```python
from build123d import *

# Parameters (mm, degrees)
SKETCH1_R                = 19.939
CIRCLE_EXTRUDE_DEPTH     = 6.35
SKETCH3_W                = 6.35
SKETCH3_H                = 39.878
RECTANGLE_EXTRUDE_DEPTH  = 127
SKETCH2_R                = 18.034
CIRCLE_CUT_DEPTH         = 129.712416732
SKETCH6_W                = 125.095
SKETCH6_H                = 36.068
RECTANGLE_CUT_DEPTH      = 129.712416732
SKETCH7_W                = 61.595
SKETCH7_H                = 36.068
END_SHAPE_DEPTH          = 6.35
SKETCH8_R                = 1.905
FOR_SPRING_EXTRUDE_DEPTH = 2.54
MIRRORED_PATTERN_COUNT   = 2
MIRRORED_PATTERN_PITCH   = 254
MIDDLE_CONNECTOR_REACH   = 256.861
SKETCH10_W               = 6.35
SKETCH10_H               = 39.878
SKETCH11_W               = 6.35
SKETCH11_H               = 39.878
END_CUT_DEPTH            = 55.88


with BuildPart() as part:
    # Sketch1 → circle extrude (new body)
    with BuildSketch(Plane.XY):
        Circle(SKETCH1_R)
    extrude(amount=CIRCLE_EXTRUDE_DEPTH)

    # Sketch3 → rectangle extrude (add)
    with BuildSketch(Plane(origin=(0, 0, 0), x_dir=(0, 0, -1), z_dir=(1, 0, 0))):
        with Locations((-3.175, 0)):
            Rectangle(SKETCH3_W, SKETCH3_H)
    extrude(amount=RECTANGLE_EXTRUDE_DEPTH)

    # Sketch2 → circle cut (cut, through all)
    with BuildSketch(Plane.XY.offset(6.35)):
        Circle(SKETCH2_R)
    extrude(amount=-CIRCLE_CUT_DEPTH, mode=Mode.SUBTRACT)

    # Sketch6 → rectangle cut (cut, through all)
    with BuildSketch(Plane.XY.offset(6.35)):
        with Locations((62.5475, 0)):
            Rectangle(SKETCH6_W, SKETCH6_H)
    extrude(amount=-RECTANGLE_CUT_DEPTH, mode=Mode.SUBTRACT)

    # Sketch7 → end shape (add)
    with BuildSketch(Plane.XY.offset(6.35)):
        with Locations((94.2975, 0)):
            Rectangle(SKETCH7_W, SKETCH7_H)
    extrude(amount=-END_SHAPE_DEPTH)

    # Sketch8 → for spring extrude (add)
    with BuildSketch(Plane.ZY.offset(-63.5)):
        with Locations((3.175, 0)):
            Circle(SKETCH8_R)
    extrude(amount=FOR_SPRING_EXTRUDE_DEPTH)


with BuildPart() as mirrored_pattern_1:
    # mirrored pattern: pattern copy
    add(part.part.moved(Location(Vector(1, 0, 0) * (1 * MIRRORED_PATTERN_PITCH))))

    # Sketch10 → middle connector (add, up to next)
    with BuildSketch(Plane(origin=(127, 0, 0), x_dir=(0, 0, -1), z_dir=(1, 0, 0)), mode=Mode.PRIVATE) as middle_connector_sk1:
        with Locations((-3.175, 0)):
            Rectangle(SKETCH10_W, SKETCH10_H)
    middle_connector_tool1 = extrude(middle_connector_sk1.sketch, amount=MIDDLE_CONNECTOR_REACH, mode=Mode.PRIVATE) - mirrored_pattern_1.part

    add(part.part)  # middle connector merges part
    add(middle_connector_tool1.solids().sort_by_distance((127, 0, 3.175))[0])

    # Sketch11 → end cut (cut)
    with BuildSketch(Plane(origin=(381, 0, 0), x_dir=(0, 0, -1), z_dir=(1, 0, 0))):
        with Locations((-3.175, 0)):
            Rectangle(SKETCH11_W, SKETCH11_H)
    extrude(amount=-END_CUT_DEPTH, mode=Mode.SUBTRACT)


solid = mirrored_pattern_1.part
```
The model under review builds one solid part; all positions refer to its coordinate system, in mm. A direction names the side the tool comes from. Round coordinates to 2 decimals unless told otherwise and drop trailing zeros. Order: outer loops, then holes, each group sorted by start corner. A loop starts at its lowest first (then second) coordinate and runs counter-clockwise, first axis right, second up. Notation, with made-up numbers: (40.5, 57) -> (82.5, 57) arc R33 ccw to (82.5, 91) -> close; hole circle Ø5 at (-1.5, 44.25). An arc over 180 degrees is marked (long way). One line per item, written item: value. Start each with the question number.
Q1. Machinability: for faces 1 (the face through (31, -18.034, 3)), 2 (the face through (160, 19.939, 3)), which of the approach directions +Z, -Z, +X, -X, +Y, -Y give a long, thin tool a straight path to every point of the face, cutting with its end or side? Answer none if there is none.
Q2. Take a section at C-C (z = 2.25). Write out the cut boundary in (x, y), and give its area (3 significant figures).
Q3. Mouldability with a two-part tool opening along Y and no side actions: class faces 3 (the face through (63.5, 0, 1)), 4 (the face through (150, 0, 6.35)), 5 (the face through (285, -18.034, 3)), 6 (the face through (160, -19.939, 3)) as released by +Y, released by -Y, zero draft, split by the parting line, or undercut.
Q4. Take a section at A-A (x = 44). Write out the cut boundary in (y, z), and give its area (3 significant figures).
Q5. Take a section at D-D (y = -9). Write out the cut boundary in (x, z), and give its area (3 significant figures).
Q6. Take a section at B-B (y = 9.5). Write out the cut boundary in (x, z).
Q7. Wall thickness on line 1 (X direction, y = 5.5, z = 5.25); line 2 (Y direction, x = 59, z = 3.5); line 3 (X direction, y = 14.5, z = 3): over which ranges is each line inside the solid? List them lowest first.
Q8. Clearance check with flat-ended pins moving along their axes: pin 1 Ø1.9 at (y, z) = (-0.5, 3.5) entering from -X; pin 2 Ø1.9 at (y, z) = (-6, 2) entering from -X; pin 3 Ø1.5 at (y, z) = (-9, 3) entering from -X. State where each tip first meets the part, or that it passes through.
Reported:
1. face 1: +Z, -Z
1. face 2: +Z, -Z, +X, -X, +Y
2. outline: (0, -19.94) -> (325.12, -19.94) -> (325.12, 19.94) -> (0, 19.94) arc R19.94 ccw to start; hole (0, -18.03) -> (63.5, -18.03) -> (63.5, -1.67) -> (60.96, -1.67) -> (60.96, 1.67) -> (63.5, 1.67) -> (63.5, 18.03) -> (0, 18.03) arc R18.03 ccw to start; hole (254, -18.03) -> (317.5, -18.03) -> (317.5, -1.67) -> (314.96, -1.67) -> (314.96, 1.67) -> (317.5, 1.67) -> (317.5, 18.03) -> (254, 18.03) arc R18.03 ccw to start
2. area: 8,000 mm2
3. face 3: undercut
3. face 4: zero draft
3. face 5: undercut
3. face 6: released by -Y
4. outline: (-19.94, 0) -> (-18.03, 0) -> (-18.03, 6.35) -> (-19.94, 6.35) -> close; (18.03, 0) -> (19.94, 0) -> (19.94, 6.35) -> (18.03, 6.35) -> close
4. area: 24.2 mm2
5. outline: (-17.79, 0) -> (-15.63, 0) -> (-15.63, 6.35) -> (-17.79, 6.35) -> close; (63.5, 0) -> (238.37, 0) -> (238.37, 6.35) -> (63.5, 6.35) -> close; (317.5, 0) -> (325.12, 0) -> (325.12, 6.35) -> (317.5, 6.35) -> close
5. area: 1,170 mm2
6. outline: (-17.53, 0) -> (-15.33, 0) -> (-15.33, 6.35) -> (-17.53, 6.35) -> close; (63.5, 0) -> (238.67, 0) -> (238.67, 6.35) -> (63.5, 6.35) -> close; (317.5, 0) -> (325.12, 0) -> (325.12, 6.35) -> (317.5, 6.35) -> close
7. line 1: x = -19.17 to -17.17, 63.5 to 236.83, 317.5 to 325.12
7. line 2: y = -19.94 to -18.03, 18.03 to 19.94
7. line 3: x = -13.69 to -10.72, 63.5 to 243.28, 317.5 to 325.12
8. pin 1: stops at x = -19.94
8. pin 2: stops at x = -19.29
8. pin 3: stops at x = -18.15
